Model file for the job. Use its own axes, mm. Face numbers are marked on the shaded views. A direction names the side the tool comes from. Give positions to 0.01 mm unless a question says otherwise; leave off trailing zeros. Write each loop counter-clockwise with the first axis right and the second up, starting at its lowest first coordinate (ties: lowest second). Pieces come first, ordered by that corner, then holes. Notation, with made-up numbers: (-7.5, 26) - (41.5, 26) arc R24 ccw to (41.5, 36) - close; hole circle Ø3 at (72.25, 22). An arc over 180 degrees is marked (long way). Use a Markdown table: item, result. Add a question column.
Autodesk Inventor part; units mm, degrees
ref_plane "YZ Plane" through (0, 0, 0) normal (1, 0, 0) x (0, 1, 0)
ref_plane "XZ Plane" through (0, 0, 0) normal (0, 1, 0) x (-1, 0, 0)
ref_plane "XY Plane" through (0, 0, 0) normal (0, 0, 1) x (1, 0, 0)
sketch "Skizze1" plane through (0, 0, 0) normal (0, 0, 1) x (1, 0, 0)
  line L0 (-25.5765, 16.0824) -> (54.4235, 16.0824)
  line L1 (54.4235, 16.0824) -> (54.4235, -23.9176)
  line L2 (54.4235, -23.9176) -> (-25.5765, -23.9176)
  line L3 (-25.5765, -23.9176) -> (-25.5765, 16.0824)
  line L4 (-24.3765, 14.8824) -> (53.2235, 14.8824)
  line L5 (53.2235, 14.8824) -> (53.2235, -22.7176)
  line L6 (53.2235, -22.7176) -> (-24.3765, -22.7176)
  line L7 (-24.3765, -22.7176) -> (-24.3765, 14.8824)
  point P0 (0, 0)
  dimension "d0" = 80
  dimension "d1" = 40
  dimension "d2" = 1.2
  dimension "d3" = 1.2
  dimension "d4" = 1.2
  dimension "d5" = 1.2
extrude "Extrusion1" add sketch "Skizze1" along normal blind 1 contours L4 L5 L6 L7
extrude "Extrusion2" add sketch "Skizze1" along normal blind 20
sketch "Skizze2" plane through (0, 0, 1) normal (0, 0, 1) x (1, 0, 0)
  line L0 (-24.3765, 14.8824) -> (53.2235, 14.8824)
  line L1 (-21.8265, 14.8824) -> (50.6735, 14.8824)
  line L2 (50.6735, 14.8824) -> (50.6735, -5.6176)
  line L3 (50.6735, -5.6176) -> (-21.8265, -5.6176)
  line L4 (-21.8265, -5.6176) -> (-21.8265, 14.8824)
  line L5 (-24.3765, -22.7176) -> (-24.3765, 14.8824)
  line L6 (53.2235, 14.8824) -> (53.2235, -22.7176)
  line L7 (-14.0765, 13.8824) -> (42.9235, 13.8824)
  line L8 (42.9235, 13.8824) -> (42.9235, -6.1176)
  line L9 (42.9235, -6.1176) -> (-14.0765, -6.1176)
  line L10 (-14.0765, -6.1176) -> (-14.0765, 13.8824)
  line L11 (-8.0765, -6.1176) -> (36.9235, -6.1176)
  line L12 (36.9235, -6.1176) -> (36.9235, 3.8824)
  line L13 (36.9235, 3.8824) -> (-8.0765, 3.8824)
  line L14 (-8.0765, 3.8824) -> (-8.0765, -6.1176)
  circle A0 centre (40.3835, -0.1176) radius 1
  circle A1 centre (-11.5365, -0.1176) radius 1
  point P0 (0, 0)
  point P1 (-21.8265, 4.6324)
  point P2 (50.6735, 4.6324)
  point P3 (-14.0765, -5.6176)
  point P4 (-8.0765, -5.6176)
  point P5 (36.9235, -5.6176)
  point P6 (42.9235, -5.6176)
  dimension "d10" = 20.5
  dimension "d11" = 72.5
  dimension "d12" = 2.55
  dimension "d13" = 2.55
  dimension "d14" = 1
  dimension "d15" = 57
  dimension "d16" = 7.75
  dimension "d17" = 20
  dimension "d18" = 2
  dimension "d19" = 2
  dimension "d20" = 2.54
  dimension "d21" = 2.54
  dimension "d25" = 14
  dimension "d26" = 14
  dimension "d27" = 10
  dimension "d28" = 6
  dimension "d29" = 6
extrude "Extrusion3" add sketch "Skizze2" along normal blind 5.5 contours L10 L7 L8 L3 L12 L13 L14
sketch "Skizze3" plane through (54.4235, -23.9176, 0) normal (1, 0, 0) x (0, 0, -1)
  circle A0 centre (-17, 17) radius 1
  line L0 (0, 40) -> (-20, 40)
  line L1 (-20, 0) -> (-20, 40)
  circle A1 centre (-12.7552, 8.7755) radius 3
  point P0 (0, 23.9176)
  dimension "d32" = 2
  dimension "d33" = 23
  dimension "d34" = 3
  dimension "d35" = 6
extrude "Extrusion4" cut sketch "Skizze3" against normal through all contours A0
extrude "Extrusion5" cut sketch "Skizze3" against normal blind 1.2 contours A1
sketch "Skizze4" plane through (-25.5765, -23.9176, 0) normal (0, -1, 0) x (1, 0, 0)
  line L0 (78.8, 1) -> (1.2, 1)
  line L1 (37.5, 1) -> (42.5, 1)
  line L2 (42.5, 1) -> (42.5, 4)
  line L3 (42.5, 4) -> (37.5, 4)
  line L4 (37.5, 4) -> (37.5, 1)
  line L5 (0, 0) -> (0, 20)
  line L6 (80, 0) -> (80, 20)
  point P0 (25.5765, 0)
  point P1 (37.5, 2.5)
  point P2 (42.5, 2.5)
  dimension "d40" = 5
  dimension "d41" = 3
  dimension "d42" = 37.5
  dimension "d43" = 37.5
extrude "Extrusion6" cut sketch "Skizze4" against normal blind 1.2
properties part number "Konsole"
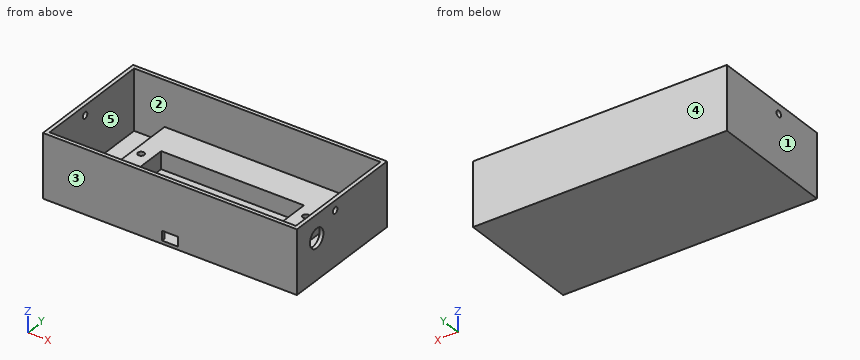
(1) Two-plate mould, pull along X, no slides. Class the marked faces 1, 2 and 3: +X half, -X half, draft (parallel to the pull), parting line (faces both ways), or undercut.
(2) Band-saw the part on D-D (y = -21). Write the cut outline in (x, z), then the cut area to 3 significant figures.
(3) Band-saw the part on A-A (z = 17). Write the cut outline in (x, y).
(4) Probe probe 1 along X at (y, z) = (4, 1.5); probe 2 along Y at (x, z) = (19, 6); probe 3 along Y at (x, z) = (-24.8, 17). List the from-to ranges inside material, lowest first. Write a range as [from, to].
(5) Which spindle directions (+Z, -Z, +X, -X, +Y, -Y) get a long thin tool onto all of the face, cutting with end or side? Do the marked faces 4 and 5. Say none if no direction does.
(6) Band-saw the part on B-B (y = -14). Write the cut outline in (x, z).
(7) Flat gauge pins, fed straight in: pin 1 (1 mm diameter, centred on x = 2.5, y = -2.5, fed in from +Z); pin 2 (2 mm diameter, centred on x = 40, y = 0, fed in from +Z). Where does each tip first touch, or does it go through?
(8) Band-saw the part on C-C (x = 36). Write the cut outline in (y, z).
Model answer:
| question | item | result |
|---|---|---|
| 1 | face 1 | -X half |
| 1 | face 2 | undercut |
| 1 | face 3 | draft |
| 2 | outline | (-25.58, 0) - (54.42, 0) - (54.42, 20) - (53.22, 20) - (53.22, 1) - (-24.38, 1) - (-24.38, 20) - (-25.58, 20) - close |
| 2 | area | 126 mm^2 |
| 3 | outline | (-25.58, -23.92) - (54.42, -23.92) - (54.42, -7.92) - (53.22, -7.92) - (53.22, -22.72) - (-24.38, -22.72) - (-24.38, -7.92) - (-25.58, -7.92) - close; (-25.58, -5.92) - (-24.38, -5.92) - (-24.38, 14.88) - (53.22, 14.88) - (53.22, -5.92) - (54.42, -5.92) - (54.42, 16.08) - (-25.58, 16.08) - close |
| 4 | probe 1 | x = [-25.58, -24.38], [-14.08, 42.92], [53.22, 54.42] |
| 4 | probe 2 | y = [-23.92, -22.72], [3.88, 13.88], [14.88, 16.08] |
| 4 | probe 3 | y = [-23.92, -7.92], [-5.92, 16.08] |
| 5 | face 4 | +Z, -Z, +X, -X, +Y |
| 5 | face 5 | +Z |
| 6 | outline | (-25.58, 0) - (54.42, 0) - (54.42, 9.98) - (53.22, 9.98) - (53.22, 1) - (-24.38, 1) - (-24.38, 20) - (-25.58, 20) - close; (53.22, 15.53) - (54.42, 15.53) - (54.42, 20) - (53.22, 20) - close |
| 7 | pin 1 | stops at z = 1 |
| 7 | pin 2 | stops at z = 6.5 |
| 8 | outline | (-23.92, 0) - (16.08, 0) - (16.08, 20) - (14.88, 20) - (14.88, 1) - (13.88, 1) - (13.88, 6.5) - (3.88, 6.5) - (3.88, 1) - (-22.72, 1) - (-22.72, 20) - (-23.92, 20) - close |
